The listing builds one solid part. Answer for the finished solid, in the listing's coordinates (mm). Face numbers are marked on the shaded views. A direction names the side the tool comes from. Coordinates: 2 decimals unless noted, no trailing zeros. Write each loop counter-clockwise with the first axis right and the second up, starting at its lowest first coordinate (ties: lowest second). Pieces come first, ordered by that corner, then holes. Notation, with made-up numbers: M 85.5,-2 L 136.5,-2 A21 ccw 136.5,30 Z; hole C 65.25,72 d4. An arc over 180 degrees is marked long. Put each result on its own line as item: value. Start each with the question number.
```python
from build123d import *

# Parameters (mm, degrees)
SKETCH1_W               = 20
SKETCH1_H               = 30
BOSS_EXTRUDE1_DEPTH     = 25
SKETCH2_W               = 20
SKETCH2_H               = 7
SKETCH2_H_2             = 6.997545124
CUT_EXTRUDE1_DEPTH      = 20
SKETCH3_W               = 5
SKETCH3_H               = 30
BOSS_EXTRUDE3_DEPTH     = 20
CUT_EXTRUDE2_DEPTH      = 13
CUT_EXTRUDE2_DEPTH_BACK = 16
SKETCH5_R               = 2.5
FILLET1_R               = 9
CUT_EXTRUDE3_DEPTH      = 11
CUT_EXTRUDE3_DEPTH_BACK = 33
SKETCH6_R               = 2
FILLET2_R               = 2
FILLET3_R               = 2
FILLET4_R               = 2


with BuildPart() as part:
    # Sketch1 → Boss-Extrude1 (new body)
    with BuildSketch(Plane.XY):
        Rectangle(SKETCH1_W, SKETCH1_H)
    extrude(amount=BOSS_EXTRUDE1_DEPTH)

    # Sketch2 → Cut-Extrude1 (cut)
    with BuildSketch(Plane(origin=(0, 0, 0), x_dir=(-1, 0, 0), z_dir=(0, 0, -1))):
        with Locations((0, 7)):
            Rectangle(SKETCH2_W, SKETCH2_H)
        with Locations((0, -7.001227438)):
            Rectangle(SKETCH2_W, SKETCH2_H_2)
    extrude(amount=-CUT_EXTRUDE1_DEPTH, mode=Mode.SUBTRACT)

    # Sketch3 → Boss-Extrude3 (add)
    with BuildSketch(Plane.XY.offset(25)):
        with Locations((-2.5, 0)):
            Rectangle(SKETCH3_W, SKETCH3_H)
    extrude(amount=BOSS_EXTRUDE3_DEPTH)

    # Sketch5 → Cut-Extrude2 (cut, two sides: drawn at the far end of the back side and taken through both)
    with BuildSketch(Plane(origin=(0, 0, 0), x_dir=(0, 0, -1), z_dir=(1, 0, 0)).offset(-CUT_EXTRUDE2_DEPTH_BACK)):
        with Locations(Location((-36, 0, 0), (0, 0, 270))):
            Circle(SKETCH5_R)
    extrude(amount=CUT_EXTRUDE2_DEPTH + CUT_EXTRUDE2_DEPTH_BACK, mode=Mode.SUBTRACT)

    # Fillet1
    fillet1_edges = [part.edges().sort_by_distance(p)[0] for p in [
        (10, -0.001227438, 0),
        (10, 12.75, 0),
        (-10, -0.001227438, 0),
        (-10, -12.75, 0),
        (-10, 12.75, 0),
        (10, -12.75, 0),
    ]]
    fillet(fillet1_edges, radius=FILLET1_R)

    # Sketch6 → Cut-Extrude3 (cut, two sides: drawn at the far end of the back side and taken through both)
    with BuildSketch(Plane(origin=(0, 15, 0), x_dir=(1, 0, 0), z_dir=(0, 1, 0)).offset(-CUT_EXTRUDE3_DEPTH_BACK)):
        with Locations((0, -9)):
            Circle(SKETCH6_R)
    extrude(amount=CUT_EXTRUDE3_DEPTH + CUT_EXTRUDE3_DEPTH_BACK, mode=Mode.SUBTRACT)

    # Fillet2
    fillet2_edges = [part.edges().sort_by_distance(p)[0] for p in [
        (-10, 0, 25),
        (-5, 0, 25),
    ]]
    fillet(fillet2_edges, radius=FILLET2_R)

    # Fillet3
    fillet3_edges = [part.edges().sort_by_distance(p)[0] for p in [
        (10, 0, 25),
    ]]
    fillet(fillet3_edges, radius=FILLET3_R)

    # Fillet4
    fillet4_edges = [part.edges().sort_by_distance(p)[0] for p in [
        (-5, 0, 45),
    ]]
    fillet(fillet4_edges, radius=FILLET4_R)


solid = part.part
```
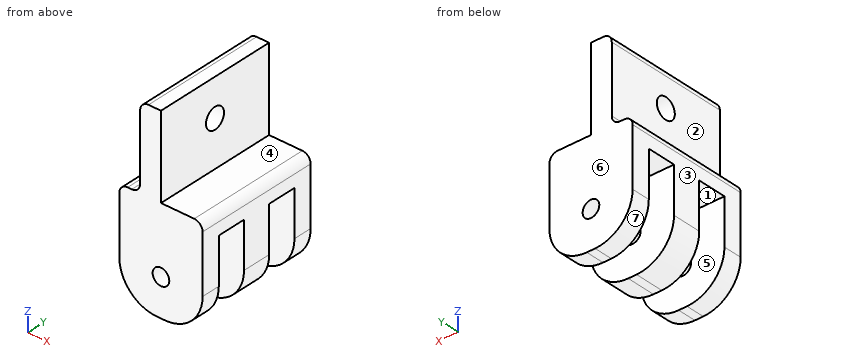
1) A cutting plane is placed at D-D on y = -5.75. Write down the section's boundary in (x, z), then the cut area to 3 significant figures.
2) A cutting plane is placed at C-C on z = 17.5. Write down the section's boundary in (x, y), then the cut area to 3 significant figures.
3) For the marked faces 1, 2, 3 and 4, determine the directions among +Z, -Z, +X, -X, +Y, -Y from which every point of the face is accessible in a straight line to the end or side of a thin tool.
4) A cutting plane is placed at B-B on z = 36. Write down the section's boundary in (x, y), then the cut area to 3 significant figures.
5) Given pin 1 Ø3.5 at (x, y) = (2.5, -7.5) entering from -Z; pin 2 Ø6 at (x, y) = (-5.5, -5) entering from -Z; pin 3 Ø8 at (y, z) = (5, 38.5) entering from -X, each flat-ended and moving along its own axis, determine where each tip first touches the part or whether it passes through.
6) A cutting plane is placed at A-A on y = 0. Write down the section's boundary in (x, z), then the cut area to 3 significant figures.
7) Straight lines are drawn through the part: probe 1 along Y at (x, z) = (-8, 9); probe 2 along Z at (x, y) = (-1.3, 0) (3 decimals); probe 3 along X at (y, z) = (-6, 36.5). For each, find the intervals that lie inside material, in ascending order.
8) Determine the mould class of the marked faces 5, 6 and 7 for opening direction Y: +Y half, -Y half, draft (parallel to the pull), parting line (faces both ways), or undercut.
Answers follow:
1. outline: M -10,20 L 10,20 L 10,23 A2 ccw 8,25 L 0,25 L 0,45 L -3,45 A2 ccw -5,43 L -5,27 A2 cw -7,25 L -8,25 A2 ccw -10,23 Z
1. area: 198 mm²
2. outline: M -10,-15 L 10,-15 L 10,-10.5 L -10,-10.5 Z; M -10,-3.5 L 10,-3.5 L 10,3.5 L -10,3.5 Z; M -10,10.5 L 10,10.5 L 10,15 L -10,15 Z
2. area: 320 mm²
3. face 1: -Z, +X, -X
3. face 2: +Z, -X, +Y, -Y
3. face 3: +Z, -Z, -X, +Y, -Y
3. face 4: +Z, +X, +Y, -Y
4. outline: M -5,-15 L 0,-15 L 0,-2.5 L -5,-2.5 Z; M -5,2.5 L 0,2.5 L 0,15 L -5,15 Z
4. area: 125 mm²
5. pin 1: stops at z = 20
5. pin 2: stops at z = 0.2
5. pin 3: stops at x = -5
6. outline: M -10,9 A9 ccw -1,0 L 1,0 A9 ccw 10,9 L 10,23 A2 ccw 8,25 L 0,25 L 0,33.5 L -5,33.5 L -5,27 A2 cw -7,25 L -8,25 A2 ccw -10,23 Z; M -5,38.5 L 0,38.5 L 0,45 L -3,45 A2 ccw -5,43 Z; hole C 0,9 d4
6. area: 526 mm²
7. probe 1: y = -15 to -10.5, -3.5 to 3.5, 10.5 to 15
7. probe 2: z = 0.005 to 7.48, 10.52 to 33.5, 38.5 to 45
7. probe 3: x = -5 to 0
8. face 5: undercut
8. face 6: +Y half
8. face 7: draft
